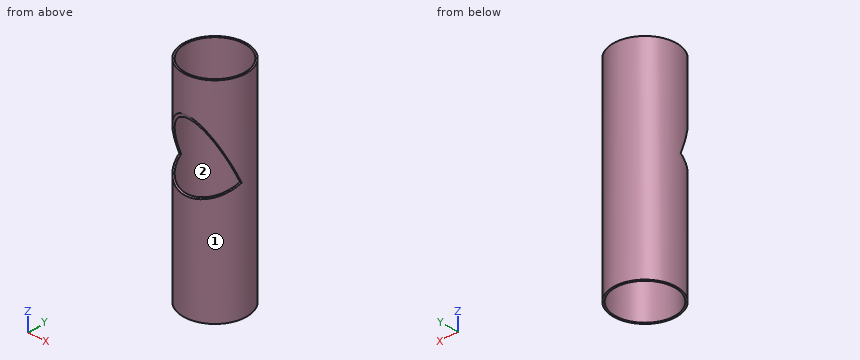
from build123d import *

# Parameters (mm, degrees)
F0_R     = 45
F1_DEPTH = 150
F2_T     = -2.5
F4_DEPTH = 50


with BuildPart() as f1:
    # F0 (on Top) → F1 (new body, symmetric)
    with BuildSketch(Plane.XY):
        Circle(F0_R)
    extrude(amount=F1_DEPTH, both=True)

    # F2
    f2_openings = [f1.faces().sort_by_distance(p)[0] for p in [
        (0, 0, 150),
        (0, 0, -150),
    ]]
    offset(amount=F2_T, openings=f2_openings)

    # F3 (on Right) → F4 (cut, symmetric)
    with BuildSketch(Plane.YZ):
        Polygon((-45, 100.388468), (-45, 0.388468), (-7, 17.892315), align=None)
    extrude(amount=F4_DEPTH, both=True, mode=Mode.SUBTRACT)


solid = f1.part
Build history of the part. All positions in model axes, mm. Face numbers are marked on the shaded views. Give positions to 0.01 mm unless a question says otherwise; leave off trailing zeros. Order: outer loops, then holes, each group sorted by start corner. A loop starts at its lowest first (then second) coordinate and runs counter-clockwise, first axis right, second up. Notation, with made-up numbers: M 6.25,41.5 L 27.25,41.5 A19 cw 27.25,65.5 Z; hole C 1,52.25 d5. An arc over 180 degrees is marked long. Put each result on its own line as item: value.
Item 1: Pull direction Y, two halves, no side cores. Call the marked faces 1 and 2: +Y half, -Y half, draft (parallel to the pull), parting line (faces both ways), or undercut.
Results are:
face 1: parting line
face 2: undercut
Item 2: Cut at D-D on z = -82. Write the cut outline in (x, y), then the cut area to 3 significant figures.
Results are:
outline: C 0,0 d90; hole C 0,0 d85
area: 687 mm2
Item 3: Cut at A-A on y = 0. Write the cut outline in (x, z), then the cut area to 3 significant figures.
Results are:
outline: M -45,-150 L -42.5,-150 L -42.5,150 L -45,150 Z; M 42.5,-150 L 45,-150 L 45,150 L 42.5,150 Z
area: 1,500 mm2
Item 4: Drop flat-ended pins along their axis: pin 1 Ø3 at (x, z) = (-22.5, 52.5) entering from +Y; pin 2 Ø12 at (x, z) = (1.5, 78) entering from -Y; pin 3 Ø12 at (x, z) = (17.5, 104.5) entering from +Y. Give the stop position or say it passes through.
Results are:
pin 1: y = 39.8
pin 2: y = 41.83
pin 3: y = 43.51
Item 5: Wall check: probe 1 along Y at (x, z) = (0, -73); probe 2 along Y at (x, z) = (0, 9); probe 3 along X at (y, z) = (-6, 94). Give the ranges that are in metal, low to high.
Results are:
probe 1: -45 to -42.5, 42.5 to 45
probe 2: 42.5 to 45
probe 3: -44.6 to -42.07, 42.07 to 44.6
Item 6: Cut at C-C on y = -24. Write the cut outline in (x, z), then the cut area to 3 significant figures.
Results are:
outline: M -38.07,-150 L -35.07,-150 L -35.07,10.06 L -38.07,10.06 Z; M -38.07,54.8 L -35.07,54.8 L -35.07,150 L -38.07,150 Z; M 35.07,-150 L 38.07,-150 L 38.07,10.06 L 35.07,10.06 Z; M 35.07,54.8 L 38.07,54.8 L 38.07,150 L 35.07,150 Z
area: 1,530 mm2
Item 7: Cut at B-B on x = -26.5. Write the cut outline in (y, z), then the cut area to 3 significant figures.
Results are:
outline: M -36.37,-150 L -33.23,-150 L -33.23,5.81 L -36.37,4.36 Z; M -36.37,81.65 L -33.23,74.83 L -33.23,150 L -36.37,150 Z; M 33.23,-150 L 36.37,-150 L 36.37,150 L 33.23,150 Z
area: 1,660 mm2
